Source: CAD feature listing. Evaluate the final solid. Frame: model axes, mm. Face numbers are marked on the shaded views. A direction names the side the tool comes from. Round coordinates to 2 decimals unless told otherwise and drop trailing zeros. Loops run counter-clockwise (first coordinate to the right, second up) from the corner with the lowest first, then second, coordinate; pieces in that order, holes last. Notation, with made-up numbers: (67, -37.5) - (118, -37.5) arc R16 cw to (118, -29.5) - close; hole circle Ø1 at (78.5, 44.25). An arc over 180 degrees is marked (long way). Write item = value, one per line. Start each with the question number.
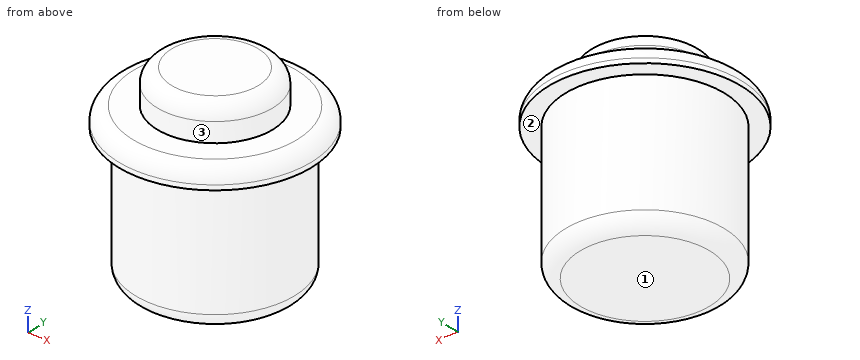
from build123d import *

# Parameters (mm, degrees)
F0_R     = 6
F1_DEPTH = 5.5
F0_R_2   = 10
F0_R_3   = 8.25
F2_DEPTH = 2
F3_DEPTH = 14
F4_R     = 1.5


with BuildPart() as f1:
    # F0 (on Top) → F1 (new body)
    with BuildSketch(Plane.XY):
        Circle(F0_R)
    extrude(amount=F1_DEPTH)

    # F0 (on Top) → F2 (join)
    with BuildSketch(Plane.XY):
        Circle(F0_R_2)
        Circle(F0_R_3, mode=Mode.SUBTRACT)
        Circle(F0_R_3)
        Circle(F0_R, mode=Mode.SUBTRACT)
    extrude(amount=F2_DEPTH)

    # F0 (on Top) → F3 (join)
    with BuildSketch(Plane.XY):
        Circle(F0_R_3)
        Circle(F0_R, mode=Mode.SUBTRACT)
        Circle(F0_R)
    extrude(amount=-F3_DEPTH)

    # F4
    f4_edges = [f1.edges().sort_by_distance(p)[0] for p in [
        (-10, 0, 2),
        (-6, 0, 5.5),
        (-8.25, 0, -14),
    ]]
    fillet(f4_edges, radius=F4_R)


solid = f1.part
(1) Cut plane D-D (z = 2.75). Output: boundary loops of the cut face in (x, y).
(2) Material intervals for line 1 along Z through (x, y) = (-1, -8.25); line 2 along Z through (x, y) = (1, 4.5); line 3 along X through (y, z) = (4.75, -0.75), sorted ascending. Write a range as from..to.
(3) Pin query (flat end, axial travel): P1, Ø3, axis at y = -5.5, z = -2.5, coming from the -X side; P2, Ø3, axis at x = -7.5, y = 8, coming from the -Z side; P3, Ø1.5, axis at y = -1, z = 2, coming from the +X side. Return the tip coordinate at first contact, or that it passes through.
(4) Access query for the marked faces 1, 2 and 3. Directions: +Z, -Z, +X, -X, +Y, -Y. A direction counts if a zero-diameter tool reaches every point of the face in a straight line with its end or side. Return the directions, or none.
(5) Cut plane C-C (z = -4.25). Output: boundary loops of the cut face in (x, y).
(6) Cut plane A-A (x = 0). Output: boundary loops of the cut face in (y, z), and give its area (3 significant figures).
Solution:
q1.outline = circle Ø12 at (0, 0)
q2.line_1 = 0..2
q2.line_2 = -14..5.5
q2.line_3 = -6.75..6.75
q3.P1 = -7.22
q3.P2 = 0
q3.P3 = 9.75
q4.face_1 = -Z, +X, -X, +Y, -Y
q4.face_2 = -Z
q4.face_3 = +Z
q5.outline = circle Ø16.5 at (0, 0)
q6.outline = (-10, 0) - (-8.25, 0) - (-8.25, -12.5) arc R1.5 ccw to (-6.75, -14) - (6.75, -14) arc R1.5 ccw to (8.25, -12.5) - (8.25, 0) - (10, 0) - (10, 0.5) arc R1.5 ccw to (8.5, 2) - (6, 2) - (6, 4) arc R1.5 ccw to (4.5, 5.5) - (-4.5, 5.5) arc R1.5 ccw to (-6, 4) - (-6, 2) - (-8.5, 2) arc R1.5 ccw to (-10, 0.5) - close
q6.area = 310 mm^2
